```python
from build123d import *

# Parameters (mm, degrees)
BOTTOM_PLATE_W                       = 120
BOTTOM_PLATE_H                       = 100
BOTTOM_PLATE_EXT_DEPTH               = 2
MIDDLE_ROW_R                         = 6
MIDDLE_ROW_CUT_DEPTH                 = 157.217796681
TOP_ROW_R                            = 8.25
TOP_ROW_R_2                          = 6.1
TOP_ROW_CUT_DEPTH                    = 157.217796681
BOTTOM_ROW_R                         = 3.55
BOTTOM_ROW_R_2                       = 6
BOTTOM_ROW_CUT_DEPTH                 = 157.217796681
PLATE_SCREWS_R                       = 1.65
PLATE_SCREWS_CUT_DEPTH               = 157.217796681
PLATE_SCREW_HEAD_R                   = 2.8
PLATE_SCREW_HEAD_CUT_DEPTH           = 2
PLATE_SCREW_HEAD_CUT_DRAFT           = -45
PLATE_SCREW_HEAD_CUT_PROFILE_2_DEPTH = 2
PLATE_SCREW_HEAD_CUT_PROFILE_2_DRAFT = -45
PLATE_SCREW_HEAD_CUT_PROFILE_3_DEPTH = 2
PLATE_SCREW_HEAD_CUT_PROFILE_3_DRAFT = -45
PLATE_SCREW_HEAD_CUT_PROFILE_4_DEPTH = 2
PLATE_SCREW_HEAD_CUT_PROFILE_4_DRAFT = -45
FILLET1_R                            = 2
FILLET2_R                            = 2
FILLET3_R                            = 2
FILLET4_R                            = 2


with BuildPart() as part:
    # Bottom Plate → Bottom Plate EXT (new body)
    with BuildSketch(Plane(origin=(0, 0, 0), x_dir=(1, 0, 0), z_dir=(0, 1, 0))):
        with Locations((-60, 50)):
            Rectangle(BOTTOM_PLATE_W, BOTTOM_PLATE_H)
    extrude(amount=BOTTOM_PLATE_EXT_DEPTH)

    # Middle Row → Middle Row Cut (cut, through all)
    with BuildSketch(Plane(origin=(0, 2, 0), x_dir=(1, 0, 0), z_dir=(0, 1, 0))):
        with Locations(Location((-105, 53, 0), (0, 0, 270))):
            Circle(MIDDLE_ROW_R)
        with Locations(Location((-75, 53, 0), (0, 0, 270))):
            Circle(MIDDLE_ROW_R)
        with Locations(Location((-45, 53, 0), (0, 0, 270))):
            Circle(MIDDLE_ROW_R)
        with Locations(Location((-15, 53, 0), (0, 0, 270))):
            Circle(MIDDLE_ROW_R)
    extrude(amount=-MIDDLE_ROW_CUT_DEPTH, mode=Mode.SUBTRACT)

    # Top Row → Top Row Cut (cut, through all)
    with BuildSketch(Plane(origin=(0, 2, 0), x_dir=(1, 0, 0), z_dir=(0, 1, 0))):
        with Locations(Location((-105, 83, 0), (0, 0, 270))):
            Circle(TOP_ROW_R)
        with Locations(Location((-75, 83, 0), (0, 0, 270))):
            Circle(TOP_ROW_R_2)
        with Locations(Location((-45, 83, 0), (0, 0, 270))):
            Circle(TOP_ROW_R_2)
        with Locations(Location((-15, 83, 0), (0, 0, 270))):
            Circle(TOP_ROW_R_2)
    extrude(amount=-TOP_ROW_CUT_DEPTH, mode=Mode.SUBTRACT)

    # Bottom Row → Bottom Row Cut (cut, through all)
    with BuildSketch(Plane(origin=(0, 2, 0), x_dir=(1, 0, 0), z_dir=(0, 1, 0))):
        with Locations(Location((-75, 20, 0), (0, 0, 270))):
            Circle(BOTTOM_ROW_R)
        with Locations(Location((-45, 20, 0), (0, 0, 270))):
            Circle(BOTTOM_ROW_R)
        with Locations(Location((-15, 20, 0), (0, 0, 270))):
            Circle(BOTTOM_ROW_R)
        with Locations(Location((-105, 20, 0), (0, 0, 270))):
            Circle(BOTTOM_ROW_R_2)
    extrude(amount=-BOTTOM_ROW_CUT_DEPTH, mode=Mode.SUBTRACT)

    # Plate Screws → Plate Screws Cut (cut, through all)
    with BuildSketch(Plane(origin=(0, 2, 0), x_dir=(1, 0, 0), z_dir=(0, 1, 0))):
        with Locations(Location((-115, 95, 0), (0, 0, 270))):
            Circle(PLATE_SCREWS_R)
        with Locations(Location((-5, 95, 0), (0, 0, 270))):
            Circle(PLATE_SCREWS_R)
        with Locations(Location((-5, 5, 0), (0, 0, 270))):
            Circle(PLATE_SCREWS_R)
        with Locations(Location((-115, 5, 0), (0, 0, 270))):
            Circle(PLATE_SCREWS_R)
    extrude(amount=-PLATE_SCREWS_CUT_DEPTH, mode=Mode.SUBTRACT)


with BuildPart() as plate_screw_head_cut_tool:
    # Plate Screw Head → Plate Screw Head Cut (with draft: the straight prism first)
    with BuildSketch(Plane(origin=(0, 2, 0), x_dir=(1, 0, 0), z_dir=(0, 1, 0))):
        with Locations((-115, 95)):
            Circle(PLATE_SCREW_HEAD_R)
    extrude(amount=-PLATE_SCREW_HEAD_CUT_DEPTH)
    # Plate Screw Head Cut: the draft: its side faces are tilted about the plane it starts from
    plate_screw_head_cut_sides = [plate_screw_head_cut_tool.faces().sort_by_distance(p)[0] for p in [
        (-117.8, 1, -95),
    ]]
    draft(plate_screw_head_cut_sides, Plane(origin=(0, 2, 0), x_dir=(1, 0, 0), z_dir=(0, 1, 0)), PLATE_SCREW_HEAD_CUT_DRAFT)


with BuildPart() as part_1:
    add(part.part)

    # Plate Screw Head Cut: cut by plate_screw_head_cut_tool
    add(plate_screw_head_cut_tool.part, mode=Mode.SUBTRACT)


with BuildPart() as plate_screw_head_cut_profile_2_tool:
    # Plate Screw Head → Plate Screw Head Cut profile 2 (with draft: the straight prism first)
    with BuildSketch(Plane(origin=(0, 2, 0), x_dir=(1, 0, 0), z_dir=(0, 1, 0))):
        with Locations((-5, 95)):
            Circle(PLATE_SCREW_HEAD_R)
    extrude(amount=-PLATE_SCREW_HEAD_CUT_PROFILE_2_DEPTH)
    # Plate Screw Head Cut profile 2: the draft: its side faces are tilted about the plane it starts from
    plate_screw_head_cut_profile_2_sides = [plate_screw_head_cut_profile_2_tool.faces().sort_by_distance(p)[0] for p in [
        (-7.8, 1, -95),
    ]]
    draft(plate_screw_head_cut_profile_2_sides, Plane(origin=(0, 2, 0), x_dir=(1, 0, 0), z_dir=(0, 1, 0)), PLATE_SCREW_HEAD_CUT_PROFILE_2_DRAFT)


with BuildPart() as part_2:
    add(part_1.part)

    # Plate Screw Head Cut profile 2: cut by plate_screw_head_cut_profile_2_tool
    add(plate_screw_head_cut_profile_2_tool.part, mode=Mode.SUBTRACT)


with BuildPart() as plate_screw_head_cut_profile_3_tool:
    # Plate Screw Head → Plate Screw Head Cut profile 3 (with draft: the straight prism first)
    with BuildSketch(Plane(origin=(0, 2, 0), x_dir=(1, 0, 0), z_dir=(0, 1, 0))):
        with Locations((-5, 5)):
            Circle(PLATE_SCREW_HEAD_R)
    extrude(amount=-PLATE_SCREW_HEAD_CUT_PROFILE_3_DEPTH)
    # Plate Screw Head Cut profile 3: the draft: its side faces are tilted about the plane it starts from
    plate_screw_head_cut_profile_3_sides = [plate_screw_head_cut_profile_3_tool.faces().sort_by_distance(p)[0] for p in [
        (-7.8, 1, -5),
    ]]
    draft(plate_screw_head_cut_profile_3_sides, Plane(origin=(0, 2, 0), x_dir=(1, 0, 0), z_dir=(0, 1, 0)), PLATE_SCREW_HEAD_CUT_PROFILE_3_DRAFT)


with BuildPart() as part_3:
    add(part_2.part)

    # Plate Screw Head Cut profile 3: cut by plate_screw_head_cut_profile_3_tool
    add(plate_screw_head_cut_profile_3_tool.part, mode=Mode.SUBTRACT)


with BuildPart() as plate_screw_head_cut_profile_4_tool:
    # Plate Screw Head → Plate Screw Head Cut profile 4 (with draft: the straight prism first)
    with BuildSketch(Plane(origin=(0, 2, 0), x_dir=(1, 0, 0), z_dir=(0, 1, 0))):
        with Locations((-115, 5)):
            Circle(PLATE_SCREW_HEAD_R)
    extrude(amount=-PLATE_SCREW_HEAD_CUT_PROFILE_4_DEPTH)
    # Plate Screw Head Cut profile 4: the draft: its side faces are tilted about the plane it starts from
    plate_screw_head_cut_profile_4_sides = [plate_screw_head_cut_profile_4_tool.faces().sort_by_distance(p)[0] for p in [
        (-117.8, 1, -5),
    ]]
    draft(plate_screw_head_cut_profile_4_sides, Plane(origin=(0, 2, 0), x_dir=(1, 0, 0), z_dir=(0, 1, 0)), PLATE_SCREW_HEAD_CUT_PROFILE_4_DRAFT)


with BuildPart() as part_4:
    add(part_3.part)

    # Plate Screw Head Cut profile 4: cut by plate_screw_head_cut_profile_4_tool
    add(plate_screw_head_cut_profile_4_tool.part, mode=Mode.SUBTRACT)

    # Fillet1
    fillet1_edges = [part_4.edges().sort_by_distance(p)[0] for p in [
        (-120, 1, -100),
    ]]
    fillet(fillet1_edges, radius=FILLET1_R)

    # Fillet2
    fillet2_edges = [part_4.edges().sort_by_distance(p)[0] for p in [
        (0, 1, -100),
    ]]
    fillet(fillet2_edges, radius=FILLET2_R)

    # Fillet3
    fillet3_edges = [part_4.edges().sort_by_distance(p)[0] for p in [
        (0, 1, 0),
    ]]
    fillet(fillet3_edges, radius=FILLET3_R)

    # Fillet4
    fillet4_edges = [part_4.edges().sort_by_distance(p)[0] for p in [
        (-120, 1, 0),
    ]]
    fillet(fillet4_edges, radius=FILLET4_R)


solid = part_4.part
```
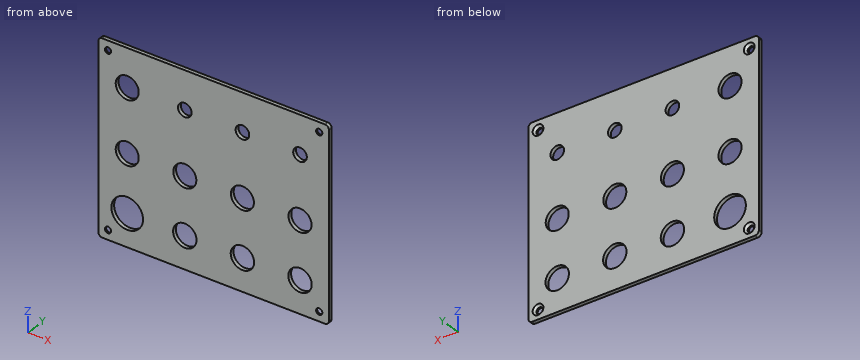
Read the model definition and answer for the solid it produces. Units are mm, in the model's axes. Round coordinates to 2 decimals unless told otherwise and drop trailing zeros. Write each loop counter-clockwise with the first axis right and the second up, starting at its lowest first coordinate (ties: lowest second). Pieces come first, ordered by that corner, then holes. Notation, with made-up numbers: (23.25, -16.5) - (61.25, -16.5) arc R9 ccw to (61.25, 0.5) - close; hole circle Ø3 at (5.5, 22). An arc over 180 degrees is marked (long way). One line per item, written item: value.
Q1. Find section B-B (z = -53). Determine the outline of the cut face in (x, y).
The answers:
outline: (-120, 0) - (-111, 0) - (-111, 2) - (-120, 2) - close; (-99, 0) - (-81, 0) - (-81, 2) - (-99, 2) - close; (-69, 0) - (-51, 0) - (-51, 2) - (-69, 2) - close; (-39, 0) - (-21, 0) - (-21, 2) - (-39, 2) - close; (-9, 0) - (0, 0) - (0, 2) - (-9, 2) - close
Q2. Each of these flat-tipped pins is pushed along its axis until it touches: P1, Ø5.5, axis at x = -45, z = -20, coming from the +Y side; P2, Ø5.5, axis at x = -115, z = -95, coming from the +Y side. Where does it stop, or does it pass through?
The answers:
P1: passes through
P2: stops at y = 1.95
Q3. Find section A-A (x = -75). Determine the outline of the cut face in (y, z).
The answers:
outline: (0, -100) - (2, -100) - (2, -89.1) - (0, -89.1) - close; (0, -76.9) - (2, -76.9) - (2, -59) - (0, -59) - close; (0, -47) - (2, -47) - (2, -23.55) - (0, -23.55) - close; (0, -16.45) - (2, -16.45) - (2, 0) - (0, 0) - close
Q4. Straight lines are drawn through the part: line 1 (X direction, y = 1.65, z = -20); line 2 (Z direction, x = -5, y = 0.35); line 3 (Z direction, x = -104.5, y = 0.65). For each, find the intervals that lie inside material, in ascending order. Write a range as from..to.
The answers:
line 1: x = -120..-111, -99..-78.55, -71.45..-48.55, -41.45..-18.55, -11.45..0
line 2: z = -100..-96.65, -93.35..-6.65, -3.35..0
line 3: z = -100..-91.23, -74.77..-58.98, -47.02..-25.98, -14.02..0
Q5. Find section C-C (z = -5). Determine the outline of the cut face in (x, y).
The answers:
outline: (-120, 0) - (-116.65, 0) - (-116.65, 0.85) - (-117.8, 2) - (-120, 2) - close; (-113.35, 0) - (-6.65, 0) - (-6.65, 0.85) - (-7.8, 2) - (-112.2, 2) - (-113.35, 0.85) - close; (-3.35, 0) - (0, 0) - (0, 2) - (-2.2, 2) - (-3.35, 0.85) - close
Q6. Find section D-D (x = -115). Determine the outline of the cut face in (y, z), and give its area (3 significant figures).
The answers:
outline: (0, -100) - (2, -100) - (2, -97.8) - (0.85, -96.65) - (0, -96.65) - close; (0, -93.35) - (0.85, -93.35) - (2, -92.2) - (2, -7.8) - (0.85, -6.65) - (0, -6.65) - close; (0, -3.35) - (0.85, -3.35) - (2, -2.2) - (2, 0) - (0, 0) - close
area: 184 mm2
